The model under review builds one solid part; all positions refer to its coordinate system, in mm. A direction names the side the tool comes from. Round coordinates to 2 decimals unless told otherwise and drop trailing zeros. Loops run counter-clockwise (first coordinate to the right, second up) from the corner with the lowest first, then second, coordinate; pieces in that order, holes last. Notation, with made-up numbers: (78.25, 50) -> (92.25, 50) arc R19 cw to (92.25, 59) -> close; hole circle Ø10 at (15, 63). An arc over 180 degrees is marked (long way). Write each question's results on one line, items separated by ' | '. Start each with the question number.
Item 1: We need section D-D (x = 11). Give the boundary of the cut face in (y, z) (3 decimals).
Item 2: We need section C-C (z = 37.5). Give the boundary of the cut face in (x, y) (3 decimals).
Item 3: We need section B-B (z = -18). Give the boundary of the cut face in (x, y) (3 decimals).
Item 4: For L1, parallel to Z at x = 0, y = -36 (3 decimals); L2, parallel to X at y = -7, z = -13.5; L3, parallel to X at y = -9, z = 20.5, list the stretches that pass through material, from the lowest coordinate up. Write a range as from..to.
Item 5: Clearance check with flat-ended pins moving along their axes: pin 1 Ø6 at (x, y) = (12, -7) entering from -Z; pin 2 Ø4 at (x, y) = (83, -26) entering from +Z; pin 3 Ø21.5 at (x, y) = (56.5, -21) entering from -Z; pin 4 Ø10 at (x, z) = (41.5, 43.5) entering from -Y. State where each tip first meets the part, or that it passes through.
Item 6: Tool access review of faces 5 (the cylindrical face through (111.18, -7.08, 15.04)), 6 (the cylindrical face through (111.18, -26.13, 15.04)), 7 (the flat face through (47.583, -16.585, 35.125)), 8 (the flat face through (63, -16, 5.55)): name each direction out of +Z, -Z, +X, -X, +Y, -Y from which nothing blocks a thin tool from reaching the whole face with its end or side.
Item 7: Mouldability with a two-part tool opening along Z and no side actions: class faces 1 (the cylindrical face through (102.24, -16.58, 47.21)), 2 (the flat face through (10, -52.375, -10)), 3 (the cylindrical face through (123.301, -16.474, -31.648)), 4 (the cylindrical face through (21.199, -42.716, 6.676)) as pulls with the +Z half, pulls with the -Z half, needs draft (parallel to the pull), parting line crosses it, or undercut.
Item 8: We need section A-A (x = 126). Give the boundary of the cut face in (y, z) (3 decimals).
from build123d import *

# Parameters (mm, degrees)
F0_R     = 22.225
F1_DEPTH = 33.3248
F0_R_2   = 12.7
F2_DEPTH = 52.3748
F4_DEPTH = 3.175
F6_DEPTH = 3.175
F7_DEPTH = 22.225
F9_DEPTH = 11.0998


with BuildPart() as f1:
    # F0 (on Front) → F1 (new body)
    with BuildSketch(Plane.XZ):
        with BuildLine():
            ThreePointArc((21.9970452561, -12.7), (24.5345159877, -6.5740037456), (25.4, 0))
            ThreePointArc((25.4, 0), (24.5345159877, 6.5740037456), (21.9970452561, 12.7))
            ThreePointArc((21.9970452561, 12.7), (10.5332083635, 23.1130162803), (-4.8465484826, 24.9333304596))
            ThreePointArc((-4.8465484826, 24.9333304596), (-20.6785341663, -14.7498550751), (21.9970452561, -12.7))
        make_face()
        Circle(F0_R, mode=Mode.SUBTRACT)
        with BuildLine():
            ThreePointArc((21.9970452561, 12.7), (24.5345159877, 6.5740037456), (25.4, 0))
            ThreePointArc((25.4, 0), (24.5345159877, -6.5740037456), (21.9970452561, -12.7))
            Line((21.9970452561, -12.7), (44.45, -12.7))
            Line((44.45, -12.7), (113.592253257, -12.7))
            ThreePointArc((113.592253257, -12.7), (114.2376587708, 3.7745620369), (112.506165921, 20.1705882353))
            ThreePointArc((112.506165921, 20.1705882353), (111.126051049, 14.9752751807), (106.2558233698, 12.7))
            Line((106.2558233698, 12.7), (44.45, 12.7))
            Line((44.45, 12.7), (21.9970452561, 12.7))
        make_face()
        with BuildLine():
            ThreePointArc((44.45, -5.5499), (40.5256280751, -3.9243719249), (38.9001, 0))
            ThreePointArc((38.9001, 0), (40.5256280751, 3.9243719249), (44.45, 5.5499))
            Line((44.45, 5.5499), (82.55, 5.5499))
            ThreePointArc((82.55, 5.5499), (88.0999, 0), (82.55, -5.5499))
            Line((82.55, -5.5499), (44.45, -5.5499))
        make_face(mode=Mode.SUBTRACT)
        with BuildLine():
            ThreePointArc((112.506165921, 20.1705882353), (114.2376587708, 3.7745620369), (113.592253257, -12.7))
            ThreePointArc((113.592253257, -12.7), (112.9058029226, -17.7980242274), (111.99067104, -22.86))
            ThreePointArc((111.99067104, -22.86), (111.7983897902, -24.1235361825), (111.7340789334, -25.4))
            ThreePointArc((111.7340789334, -25.4), (123.1576151159, -38.0356891432), (136.8774868267, -27.94))
            ThreePointArc((136.8774868267, -27.94), (138.9294471202, 14.6526012321), (128.0371649171, 55.88))
            ThreePointArc((128.0371649171, 55.88), (113.9555393972, 63.2630335862), (103.7012522936, 51.1118625227))
            ThreePointArc((103.7012522936, 51.1118625227), (103.9343890657, 48.3581167453), (104.7576803867, 45.72))
            ThreePointArc((104.7576803867, 45.72), (109.380472839, 33.1723101625), (112.506165921, 20.1705882353))
        make_face()
        with BuildLine():
            ThreePointArc((130.6557828801, -26.67), (123.1640789334, -31.6217039467), (118.2123749867, -24.13))
            ThreePointArc((118.2123749867, -24.13), (119.9845225129, 12.6545192459), (110.5775515193, 48.26))
            ThreePointArc((110.5775515193, 48.26), (113.8574226519, 56.6198711326), (122.2172937845, 53.34))
            ThreePointArc((122.2172937845, 53.34), (132.6144722511, 13.9865739034), (130.6557828801, -26.67))
        make_face(mode=Mode.SUBTRACT)
    extrude(amount=F1_DEPTH)

    # F0 (on Front) → F2 (join)
    with BuildSketch(Plane.XZ):
        Circle(F0_R)
        Circle(F0_R_2, mode=Mode.SUBTRACT)
    extrude(amount=F2_DEPTH)

    # F3 (on face) → F4 (cut)
    with BuildSketch(Plane.XZ.offset(33.3248)):
        with BuildLine():
            ThreePointArc((21.9970452561, 12.7), (24.5345159877, 6.5740037456), (25.4, 0))
            ThreePointArc((25.4, 0), (24.5345159877, -6.5740037456), (21.9970452561, -12.7))
            Line((21.9970452561, -12.7), (113.592253257, -12.7))
            ThreePointArc((113.592253257, -12.7), (112.9058029226, -17.7980242274), (111.99067104, -22.86))
            ThreePointArc((111.99067104, -22.86), (121.8940789334, -37.8434078933), (136.8774868267, -27.94))
            ThreePointArc((136.8774868267, -27.94), (138.9294471202, 14.6526012321), (128.0371649171, 55.88))
            ThreePointArc((128.0371649171, 55.88), (111.3174226519, 62.4397422652), (104.7576803867, 45.72))
            ThreePointArc((104.7576803867, 45.72), (109.380472839, 33.1723101625), (112.506165921, 20.1705882353))
            ThreePointArc((112.506165921, 20.1705882353), (111.126051049, 14.9752751807), (106.2558233698, 12.7))
            Line((106.2558233698, 12.7), (21.9970452561, 12.7))
        make_face()
        with BuildLine():
            Line((82.55, -5.5499), (44.45, -5.5499))
            ThreePointArc((44.45, -5.5499), (38.9001, 0), (44.45, 5.5499))
            Line((44.45, 5.5499), (82.55, 5.5499))
            ThreePointArc((82.55, 5.5499), (88.0999, 0), (82.55, -5.5499))
        make_face(mode=Mode.SUBTRACT)
        with BuildLine():
            ThreePointArc((130.6557828801, -26.67), (123.1640789334, -31.6217039467), (118.2123749867, -24.13))
            ThreePointArc((118.2123749867, -24.13), (119.9845225129, 12.6545192459), (110.5775515193, 48.26))
            ThreePointArc((110.5775515193, 48.26), (113.8574226519, 56.6198711326), (122.2172937845, 53.34))
            ThreePointArc((122.2172937845, 53.34), (132.6144722511, 13.9865739034), (130.6557828801, -26.67))
        make_face(mode=Mode.SUBTRACT)
    extrude(amount=-F4_DEPTH, mode=Mode.SUBTRACT)

    # F5 (on face) → F6 (cut)
    with BuildSketch(Plane(origin=(0, 0, 0), x_dir=(-1, 0, 0), z_dir=(0, 1, 0))):
        with BuildLine():
            ThreePointArc((-21.9970452561, -12.7), (-25.4, 0), (-21.9970452561, 12.7))
            Line((-21.9970452561, 12.7), (-106.2558233698, 12.7))
            ThreePointArc((-106.2558233698, 12.7), (-111.126051049, 14.9752751807), (-112.506165921, 20.1705882353))
            ThreePointArc((-112.506165921, 20.1705882353), (-109.380472839, 33.1723101625), (-104.7576803867, 45.72))
            ThreePointArc((-104.7576803867, 45.72), (-111.3174226519, 62.4397422652), (-128.0371649171, 55.88))
            ThreePointArc((-128.0371649171, 55.88), (-138.9294471202, 14.6526012321), (-136.8774868267, -27.94))
            ThreePointArc((-136.8774868267, -27.94), (-121.8940789334, -37.8434078933), (-111.99067104, -22.86))
            ThreePointArc((-111.99067104, -22.86), (-112.9058029226, -17.7980242274), (-113.592253257, -12.7))
            Line((-113.592253257, -12.7), (-21.9970452561, -12.7))
        make_face()
        with BuildLine():
            ThreePointArc((-122.2172937845, 53.34), (-113.8574226519, 56.6198711326), (-110.5775515193, 48.26))
            ThreePointArc((-110.5775515193, 48.26), (-119.9845225129, 12.6545192459), (-118.2123749867, -24.13))
            ThreePointArc((-118.2123749867, -24.13), (-123.1640789334, -31.6217039467), (-130.6557828801, -26.67))
            ThreePointArc((-130.6557828801, -26.67), (-132.6144722511, 13.9865739034), (-122.2172937845, 53.34))
        make_face(mode=Mode.SUBTRACT)
        with BuildLine():
            Line((-82.55, 5.5499), (-44.45, 5.5499))
            ThreePointArc((-44.45, 5.5499), (-38.9001, 0), (-44.45, -5.5499))
            Line((-44.45, -5.5499), (-82.55, -5.5499))
            ThreePointArc((-82.55, -5.5499), (-88.0999, 0), (-82.55, 5.5499))
        make_face(mode=Mode.SUBTRACT)
    extrude(amount=-F6_DEPTH, mode=Mode.SUBTRACT)

    # F0 (on Front) → F7 (join)
    with BuildSketch(Plane.XZ):
        with BuildLine():
            ThreePointArc((-4.8465484826, 24.9333304596), (10.5332083635, 23.1130162803), (21.9970452561, 12.7))
            Line((21.9970452561, 12.7), (44.45, 12.7))
            Line((44.45, 12.7), (106.2558233698, 12.7))
            ThreePointArc((106.2558233698, 12.7), (111.126051049, 14.9752751807), (112.506165921, 20.1705882353))
            ThreePointArc((112.506165921, 20.1705882353), (109.380472839, 33.1723101625), (104.7576803867, 45.72))
            ThreePointArc((104.7576803867, 45.72), (103.9343890657, 48.3581167453), (103.7012522936, 51.1118625227))
            ThreePointArc((103.7012522936, 51.1118625227), (102.2030178457, 47.1688368577), (98.5648042351, 45.0344611692))
            Line((98.5648042351, 45.0344611692), (-4.8465484826, 24.9333304596))
        make_face()
    extrude(amount=F7_DEPTH)

    # F8 (on face) → F9 (cut)
    with BuildSketch(Plane(origin=(0, 0, 0), x_dir=(-1, 0, 0), z_dir=(0, 1, 0))):
        with BuildLine():
            ThreePointArc((-21.9970452561, 12.7), (-10.5332083635, 23.1130162803), (4.8465484826, 24.9333304596))
            Line((4.8465484826, 24.9333304596), (-98.5648042351, 45.0344611692))
            ThreePointArc((-98.5648042351, 45.0344611692), (-102.2030178457, 47.1688368577), (-103.7012522936, 51.1118625227))
            ThreePointArc((-103.7012522936, 51.1118625227), (-103.9343890657, 48.3581167453), (-104.7576803867, 45.72))
            ThreePointArc((-104.7576803867, 45.72), (-109.380472839, 33.1723101625), (-112.506165921, 20.1705882353))
            ThreePointArc((-112.506165921, 20.1705882353), (-111.126051049, 14.9752751807), (-106.2558233698, 12.7))
            Line((-106.2558233698, 12.7), (-21.9970452561, 12.7))
        make_face()
    extrude(amount=-F9_DEPTH, mode=Mode.SUBTRACT)


solid = f1.part
Here are the results:
1) outline: (-52.375, -19.312) -> (-33.325, -19.312) -> (-33.325, -22.895) -> (0, -22.895) -> (0, -6.347) -> (-52.375, -6.347) -> close; (-52.375, 6.347) -> (0, 6.347) -> (0, 22.895) -> (-11.1, 22.895) -> (-11.1, 28.014) -> (-22.225, 28.014) -> (-22.225, 22.895) -> (-33.325, 22.895) -> (-33.325, 19.312) -> (-52.375, 19.312) -> close
2) outline: (59.803, -22.225) -> (107.973, -22.225) -> (107.973, -30.15) -> (114.674, -30.15) -> (114.674, -3.175) -> (107.973, -3.175) -> (107.973, -11.1) -> (59.803, -11.1) -> close; (127.969, -30.15) -> (134.573, -30.15) -> (134.573, -3.175) -> (127.969, -3.175) -> close
3) outline: (-17.921, -33.325) -> (-13.037, -33.325) -> (-13.037, -52.375) -> (13.037, -52.375) -> (13.037, -33.325) -> (17.921, -33.325) -> (17.921, 0) -> (-17.921, 0) -> close; (112.874, -30.15) -> (119.3, -30.15) -> (119.3, -3.175) -> (112.874, -3.175) -> close; (132.13, -30.15) -> (138.536, -30.15) -> (138.536, -3.175) -> (132.13, -3.175) -> close
4) L1: z = -22.225..-12.7, 12.7..22.225 | L2: x = -21.52..21.52, 113.5..119.89, 132.66..139.05 | L3: x = -15..15, 112.45..118.9, 131.76..138.19
5) pin 1: stops at z = -23.75 | pin 2: stops at z = 12.7 | pin 3: stops at z = -12.7 | pin 4: passes through
6) face 5: +Y | face 6: -Y | face 7: +Z, -X, +Y, -Y | face 8: +Y, -Y
7) face 1: pulls with the +Z half | face 2: needs draft | face 3: undercut | face 4: parting line crosses it
8) outline: (-30.15, -38.003) -> (-3.175, -38.003) -> (-3.175, -31.554) -> (-30.15, -31.554) -> close; (-30.15, 43.66) -> (-3.175, 43.66) -> (-3.175, 59.111) -> (-30.15, 59.111) -> close
